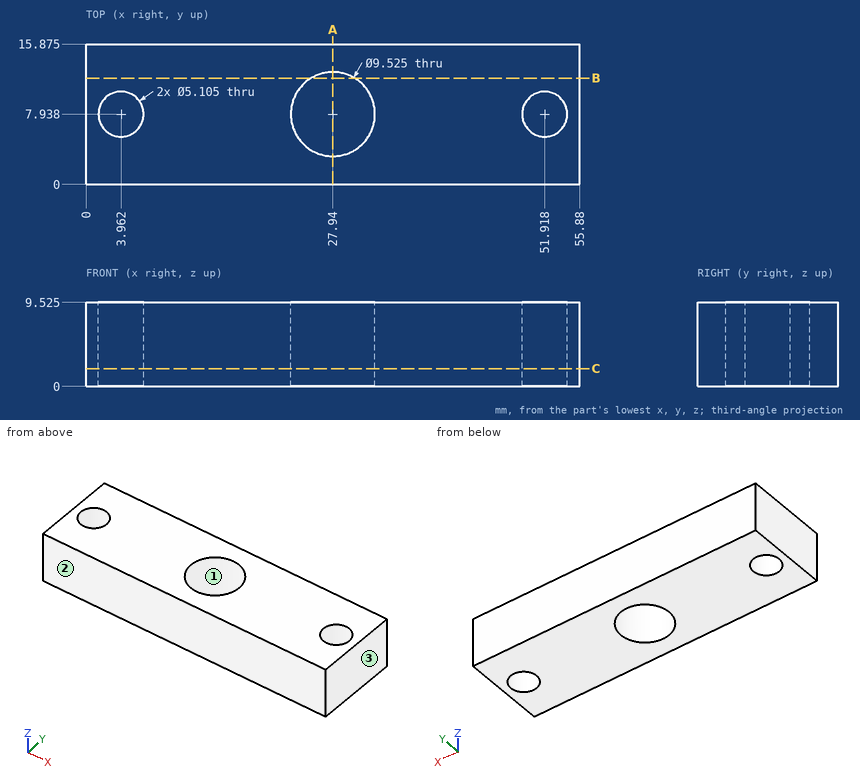
Design review of the part shown in the three views and the two pictorial views. Dimensions are in mm from the part's minimum x, y and z. Round coordinates to 2 decimals unless told otherwise and drop trailing zeros. Loops run counter-clockwise (first coordinate to the right, second up) from the corner with the lowest first, then second, coordinate; pieces in that order, holes last.
1) Wall thickness on line 1 along X through (y, z) = (6, 6) (1 decimal); line 2 along Y through (x, z) = (31, 3) (1 decimal); line 3 along Y through (x, z) = (27, 0.5) (1 decimal): over which ranges is each line inside the solid? List them lowest first.
Values follow:
line 1: x = 0 to 2.3, 5.6 to 23.6, 32.3 to 50.3, 53.6 to 55.9
line 2: y = 0 to 4.3, 11.6 to 15.9
line 3: y = 0 to 3.3, 12.6 to 15.9
2) Consider section B-B on y = 12. State the section outline as (x, z) points (1 decimal).
Values follow:
outline: (0, 0) - (25.5, 0) - (25.5, 9.5) - (0, 9.5) - close; (30.4, 0) - (55.9, 0) - (55.9, 9.5) - (30.4, 9.5) - close
3) Consider section A-A on x = 27.94. State the section outline as (y, z) points (1 decimal).
Values follow:
outline: (0, 0) - (3.2, 0) - (3.2, 9.5) - (0, 9.5) - close; (12.7, 0) - (15.9, 0) - (15.9, 9.5) - (12.7, 9.5) - close
4) Clearance check with a flat-ended pin moving along its axis: P1, Ø8.5, axis at x = 27.94, y = 7.94, coming from the +Z side. State where the tip first meets the part, or that it passes through.
Values follow:
P1: passes through
5) The part is to be moulded in two halves that separate along Y. For the marked faces 1, 2 and 3, say which applies: pulls with the +Y half, pulls with the -Y half, needs draft (parallel to the pull), parting line crosses it, or undercut.
Values follow:
face 1: undercut
face 2: pulls with the -Y half
face 3: needs draft
6) Consider section C-C on z = 2. State the section outline as (x, y) points (1 decimal).
Values follow:
outline: (0, 0) - (55.9, 0) - (55.9, 15.9) - (0, 15.9) - close; hole circle Ø5.1 at (4, 7.9); hole circle Ø9.5 at (27.9, 7.9); hole circle Ø5.1 at (51.9, 7.9)
